Here's how the part is built. I have some questions about the finished solid (model axes, mm). Coordinates: 2 decimals unless noted, no trailing zeros. Write each loop counter-clockwise with the first axis right and the second up, starting at its lowest first coordinate (ties: lowest second). Pieces come first, ordered by that corner, then holes. Notation, with made-up numbers: (5.5, 82) -> (63.5, 82) arc R11 cw to (63.5, 87) -> close; hole circle Ø8 at (42.25, 39). An arc over 180 degrees is marked (long way). Use a Markdown table: item, result. Add a question column.
```python
from build123d import *

# Parameters (mm, degrees)
F1_DEPTH = 6.35


with BuildPart() as f1:
    # F0 (on Front) → F1 (new body)
    with BuildSketch(Plane.XZ):
        with BuildLine():
            Line((-76.2, -10.16), (72.39, -10.16))
            Line((72.39, -10.16), (72.39, -5.715))
            Line((72.39, -5.715), (73.66, -5.715))
            Line((73.66, -5.715), (73.66, -6.35))
            Line((73.66, -6.35), (74.93, -6.35))
            ThreePointArc((74.93, -6.35), (76.2, -5.08), (74.93, -3.81))
            Line((74.93, -3.81), (73.66, -3.81))
            Line((73.66, -3.81), (73.66, -4.445))
            Line((73.66, -4.445), (72.39, -4.445))
            Line((72.39, -4.445), (72.39, 4.445))
            Line((72.39, 4.445), (73.66, 4.445))
            Line((73.66, 4.445), (73.66, 3.81))
            Line((73.66, 3.81), (74.93, 3.81))
            ThreePointArc((74.93, 3.81), (76.2, 5.08), (74.93, 6.35))
            Line((74.93, 6.35), (73.66, 6.35))
            Line((73.66, 6.35), (73.66, 5.715))
            Line((73.66, 5.715), (72.39, 5.715))
            Line((72.39, 5.715), (72.39, 10.16))
            Line((72.39, 10.16), (-76.2, 10.16))
            Line((-76.2, 10.16), (-76.2, 5.715))
            Line((-76.2, 5.715), (-74.93, 5.715))
            Line((-74.93, 5.715), (-74.93, 6.35))
            Line((-74.93, 6.35), (-73.66, 6.35))
            ThreePointArc((-73.66, 6.35), (-72.39, 5.08), (-73.66, 3.81))
            Line((-73.66, 3.81), (-74.93, 3.81))
            Line((-74.93, 3.81), (-74.93, 4.445))
            Line((-74.93, 4.445), (-76.2, 4.445))
            Line((-76.2, 4.445), (-76.2, -4.445))
            Line((-76.2, -4.445), (-74.93, -4.445))
            Line((-74.93, -4.445), (-74.93, -3.81))
            Line((-74.93, -3.81), (-73.66, -3.81))
            ThreePointArc((-73.66, -3.81), (-72.39, -5.08), (-73.66, -6.35))
            Line((-73.66, -6.35), (-74.93, -6.35))
            Line((-74.93, -6.35), (-74.93, -5.715))
            Line((-74.93, -5.715), (-76.2, -5.715))
            Line((-76.2, -5.715), (-76.2, -10.16))
        make_face()
    extrude(amount=F1_DEPTH)


solid = f1.part
```
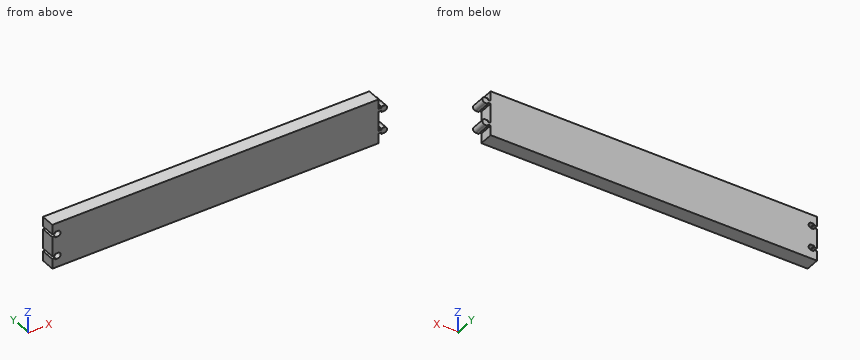
Q1. Please list where this line runs through material, in increasing order: line 1 (X direction, y = -3.75, z = 1.5).
Q2. Suppose I cut it at A-A, the plane z = -2.25. Write out the boundary of the cut face in (x, y), and give its area (3 significant figures).
Q3. Will these pins go through, and if not, where does the flat tip stop? pin 1 (1 mm diameter, centred on x = 74, y = -3, fed in from -Z); pin 2 (3 mm diameter, centred on x = 14, z = -8, fed in from +Y); pin 3 (1.3 mm diameter, centred on y = -4.5, z = 8.5, fed in from +X); pin 4 (1 mm diameter, centred on x = 73, y = -1.5, fed in from -Z) (3 decimals).
Answer key:
| question | item | result |
|---|---|---|
| 1 | line 1 | x = -76.2 to 72.39 |
| 2 | outline | (-76.2, -6.35) -> (72.39, -6.35) -> (72.39, 0) -> (-76.2, 0) -> close |
| 2 | area | 944 mm^2 |
| 3 | pin 1 | stops at z = -6.35 |
| 3 | pin 2 | stops at y = 0 |
| 3 | pin 3 | stops at x = 72.39 |
| 3 | pin 4 | stops at z = -5.715 |
